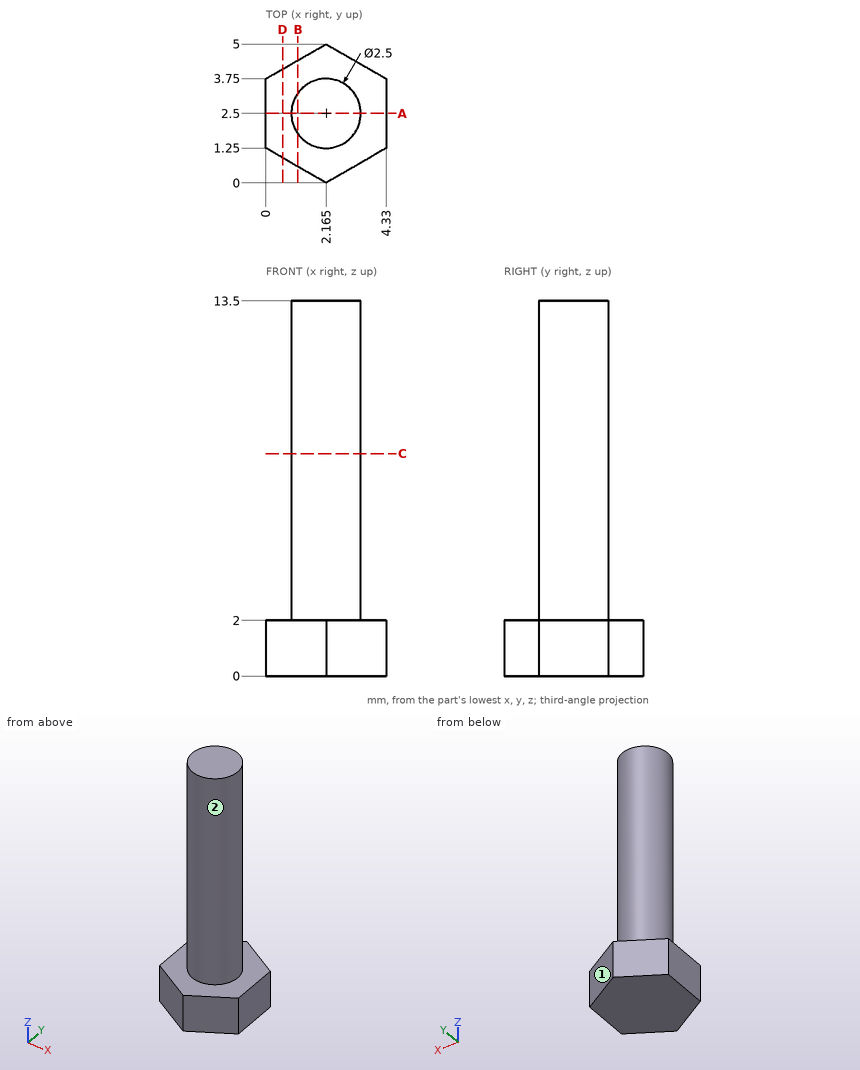
Input: dimensioned drawing with shaded views. Units: mm. Origin: part minimum x, y, z. A direction names the side the tool comes from. Give positions to 0.01 mm unless a question says otherwise; leave off trailing zeros. Write each loop counter-clockwise with the first axis right and the second up, starting at its lowest first coordinate (ties: lowest second). Pieces come first, ordered by that corner, then holes. Notation, with made-up numbers: (8, -36) -> (66, -36) arc R12 cw to (66, -13) -> close; hole circle Ø1 at (-21.5, 40). An arc over 180 degrees is marked (long way). Answer as a JSON object with one key per item and string values.
1. Access query for the marked faces 1 and 2. Directions: +Z, -Z, +X, -X, +Y, -Y. A direction counts if a zero-diameter tool reaches every point of the face in a straight line with its end or side. Return the directions, or none.
Ans:
{"face 1": "+Z, -Z, +X, +Y", "face 2": "+Z"}
2. Contact query for flat-ended pins moving along their axis: pin 1 (2 mm diameter, centred on y = 1, z = 8, fed in from -X); pin 2 (3 mm diameter, centred on y = 2, z = 8.5, fed in from -X) (3 decimals); pin 3 (1 mm diameter, centred on x = 2.5, z = 4.5, fed in from +Y). Output: stop coordinate, or through.
Ans:
{"pin 1": "stops at x = 1.02", "pin 2": "stops at x = 0.915", "pin 3": "stops at y = 3.75"}
3. Cut plane C-C on z = 8. Output: boundary loops of the cut face in (x, y) (3 decimals).
Ans:
{"outline": "circle Ø2.5 at (2.165, 2.5)"}
4. Cut plane B-B on x = 1.15. Output: boundary loops of the cut face in (y, z).
Ans:
{"outline": "(0.59, 0) -> (4.41, 0) -> (4.41, 2) -> (3.23, 2) -> (3.23, 13.5) -> (1.77, 13.5) -> (1.77, 2) -> (0.59, 2) -> close"}
5. Cut plane D-D on x = 0.6. Output: boundary loops of the cut face in (y, z).
Ans:
{"outline": "(0.9, 0) -> (4.1, 0) -> (4.1, 2) -> (0.9, 2) -> close"}
6. Cut plane A-A on y = 2.5. Output: boundary loops of the cut face in (x, z) (3 decimals), and give its area (3 significant figures).
Ans:
{"outline": "(0, 0) -> (4.33, 0) -> (4.33, 2) -> (3.415, 2) -> (3.415, 13.5) -> (0.915, 13.5) -> (0.915, 2) -> (0, 2) -> close", "area": "37.4 mm^2"}
7. Ray query, probe 1 along Z at (x, y) = (1.75, 4); probe 2 along Y at (x, z) = (2.15, 8.75); probe 3 along Y at (x, z) = (0.45, 1). Return the intervals inside material, ascending. Write a range as from..to.
Ans:
{"probe 1": "z = 0..2", "probe 2": "y = 1.25..3.75", "probe 3": "y = 0.99..4.01"}
